from build123d import *

# Parameters (mm, degrees)
SKETCH1_W                  = 70
SKETCH1_H                  = 35
BOSS_EXTRUDE1_DEPTH        = 2
SKETCH2_R                  = 3.75
BOSS_EXTRUDE2_DEPTH        = 8
SKETCH6_W                  = 70
SKETCH6_H                  = 2
BOSS_EXTRUDE3_DEPTH        = 2
F_4_3_4_3_DIAMETER_HOLE1_D = 4.3
CHAMFER1_SIZE              = 0.75
SKETCH5_W                  = 23
SKETCH5_H                  = 14
CUT_EXTRUDE1_DEPTH         = 79.89866919
SKETCH7_W                  = 27
SKETCH7_H                  = 2
SKETCH7_W_2                = 20
BOSS_EXTRUDE4_DEPTH        = 3
SKETCH9_W                  = 27
SKETCH9_H                  = 10
SKETCH9_W_2                = 20
BOSS_EXTRUDE5_DEPTH        = 3
BOSS_EXTRUDE6_DEPTH        = 20
BOSS_EXTRUDE7_START        = -43
BOSS_EXTRUDE7_DEPTH        = 27
CHAMFER3_SIZE              = 0.75
SKETCH11_W                 = 6
SKETCH11_H                 = 10
BOSS_EXTRUDE8_DEPTH        = 10
SKETCH12_R                 = 4.15
CUT_EXTRUDE2_DEPTH         = 5.2
CHAMFER4_SIZE              = 0.4


with BuildPart() as part:
    # Sketch1 → Boss-Extrude1 (new body)
    with BuildSketch(Plane(origin=(0, 0, 0), x_dir=(1, 0, 0), z_dir=(0, 1, 0))):
        with Locations((35, 17.5)):
            Rectangle(SKETCH1_W, SKETCH1_H)
    extrude(amount=BOSS_EXTRUDE1_DEPTH)

    # Sketch2 → Boss-Extrude2 (add)
    with BuildSketch(Plane(origin=(0, 2, 0), x_dir=(1, 0, 0), z_dir=(0, 1, 0))):
        with Locations(Location((66, 31, 0), (0, 0, 90))):
            Circle(SKETCH2_R)
        with Locations(Location((15, 31, 0), (0, 0, 90))):
            Circle(SKETCH2_R)
        with Locations(Location((15, 4, 0), (0, 0, 90))):
            Circle(SKETCH2_R)
        with Locations(Location((66, 4, 0), (0, 0, 90))):
            Circle(SKETCH2_R)
    extrude(amount=BOSS_EXTRUDE2_DEPTH)

    # Sketch6 → Boss-Extrude3 (add)
    with BuildSketch(Plane.XY):
        with Locations((35, 1)):
            Rectangle(SKETCH6_W, SKETCH6_H)
    extrude(amount=BOSS_EXTRUDE3_DEPTH)

    # Ø4.3 (4.3) Diameter Hole1 (through all)
    with Locations(Plane(origin=(0, 10, 0), x_dir=(1, 0, 0), z_dir=(0, 1, 0))):
        with Locations((66, 31), (15, 31), (15, 4), (66, 4)):
            Hole(F_4_3_4_3_DIAMETER_HOLE1_D / 2)

    # Chamfer1
    chamfer1_edges = [part.edges().sort_by_distance(p)[0] for p in [
        (66, 10, -27.25),
        (15, 10, -27.25),
        (15, 10, -0.25),
        (66, 10, -0.25),
    ]]
    chamfer(chamfer1_edges, length=CHAMFER1_SIZE)

    # Sketch5 → Cut-Extrude1 (cut, through all)
    with BuildSketch(Plane.XZ):
        with Locations((38.5, -5)):
            Rectangle(SKETCH5_W, SKETCH5_H)
    extrude(amount=-CUT_EXTRUDE1_DEPTH, mode=Mode.SUBTRACT)

    # Sketch7 → Boss-Extrude4 (add)
    with BuildSketch(Plane.XY.offset(2)):
        with Locations((13.5, 1)):
            Rectangle(SKETCH7_W, SKETCH7_H)
        with Locations((60, 1)):
            Rectangle(SKETCH7_W_2, SKETCH7_H)
    extrude(amount=BOSS_EXTRUDE4_DEPTH)

    # Sketch9 → Boss-Extrude5 (add)
    with BuildSketch(Plane.XY.offset(5)):
        with Locations((13.5, 5)):
            Rectangle(SKETCH9_W, SKETCH9_H)
        with Locations((60, 5)):
            Rectangle(SKETCH9_W_2, SKETCH9_H)
    extrude(amount=BOSS_EXTRUDE5_DEPTH)

    # Sketch10 → Boss-Extrude6 (add)
    with BuildSketch(Plane(origin=(70, 0, 0), x_dir=(0, 0, -1), z_dir=(1, 0, 0))):
        Polygon((-8, 7), (-11, 10), (-11, 0), (-8, 3), align=None)
    extrude(amount=-BOSS_EXTRUDE6_DEPTH)

    # Sketch10<2> → Boss-Extrude7 (add)
    with BuildSketch(Plane(origin=(70, 0, 0), x_dir=(0, 0, -1), z_dir=(1, 0, 0)).offset(BOSS_EXTRUDE7_START)):
        Polygon((-8, 7), (-11, 10), (-11, 0), (-8, 3), align=None)
    extrude(amount=-BOSS_EXTRUDE7_DEPTH)

    # Chamfer3
    chamfer3_edges = [part.edges().sort_by_distance(p)[0] for p in [
        (70, 8.5, 9.5),
        (70, 5, 11),
        (70, 1.5, 9.5),
        (27, 8.5, 9.5),
        (27, 5, 11),
        (27, 1.5, 9.5),
    ]]
    chamfer(chamfer3_edges, length=CHAMFER3_SIZE)

    # Sketch11 → Boss-Extrude8 (add)
    with BuildSketch(Plane.ZY):
        with Locations((8, 5)):
            Rectangle(SKETCH11_W, SKETCH11_H)
    extrude(amount=BOSS_EXTRUDE8_DEPTH)

    # Sketch12 → Cut-Extrude2 (cut)
    with BuildSketch(Plane.XY.offset(11)):
        with Locations((-5, 5)):
            Circle(SKETCH12_R)
    extrude(amount=-CUT_EXTRUDE2_DEPTH, mode=Mode.SUBTRACT)

    # Chamfer4
    chamfer4_edges = [part.edges().sort_by_distance(p)[0] for p in [
        (-9.15, 5, 11),
    ]]
    chamfer(chamfer4_edges, length=CHAMFER4_SIZE)


solid = part.part
Verification items for the finished model (mm, model axes). A direction names the side the tool comes from. Coordinates: 2 decimals unless noted, no trailing zeros. Write each loop counter-clockwise with the first axis right and the second up, starting at its lowest first coordinate (ties: lowest second). Pieces come first, ordered by that corner, then holes. Notation, with made-up numbers: M -18.5,-38.5 L 25.5,-38.5 A23 cw 25.5,-2.5 Z; hole C 46,-6 d10. An arc over 180 degrees is marked long. Use a Markdown table: item, result.
Q1. Sectioned sample at B-B, the plane z = -31. Record the boundary of the cut face in (x, y), plus the area to 3 significant figures.
Reply:
| item | result |
|---|---|
| outline | M 0,0 L 12.85,0 L 12.85,10 L 12,10 L 11.25,9.25 L 11.25,2 L 0,2 Z; M 17.15,0 L 63.85,0 L 63.85,10 L 63,10 L 62.25,9.25 L 62.25,2 L 18.75,2 L 18.75,9.25 L 18,10 L 17.15,10 Z; M 68.15,0 L 70,0 L 70,2 L 69.75,2 L 69.75,9.25 L 69,10 L 68.15,10 Z |
| area | 173 mm² |
Q2. Go/stop test with flat-tipped pins: P1, Ø1.5, axis at y = 2, z = 9.5, coming from the +X side; P2, Ø0.6, axis at x = 44, y = 1, coming from the +Z side; P3, Ø2.5, axis at x = -6, y = 5.5, coming from the +Z side; P4, Ø0.9, axis at y = 8.5, z = 9.5, coming from the +X side. Record where each tip stops, or that it passes through.
Reply:
| item | result |
|---|---|
| P1 | stops at x = 70 |
| P2 | stops at z = -12 |
| P3 | stops at z = 5.8 |
| P4 | stops at x = 69.7 |
Q3. Draft check along Z on faces 1 (the face through (17.282, 5.574, -28.024)), 2 (the face through (70, 1, -7)), 3 (the face through (60, 5, 11)). Enter one of: +Z half, -Z half, draft (parallel to the pull), parting line (faces both ways), or undercut.
Reply:
| item | result |
|---|---|
| face 1 | undercut |
| face 2 | draft |
| face 3 | +Z half |
Q4. Set-up check for faces 4 (the face through (27, 1.6, 3.2)), 5 (the face through (17, 10, -5.3)), 6 (the face through (0, 1, 9)), 7 (the face through (62.282, 5.574, -3.512)): record each of +Z, -Z, +X, -X, +Y, -Y from which the full face is reachable in a straight line by a thin tool's end or side.
Reply:
| item | result |
|---|---|
| face 4 | +Z, +Y, -Y |
| face 5 | +Z, -Z, +X, -X, +Y |
| face 6 | +X, -Y |
| face 7 | +Y |
Q5. Sectioned sample at D-D, the plane z = -10.5. Record the boundary of the cut face in (x, y).
Reply:
| item | result |
|---|---|
| outline | M 0,0 L 27,0 L 27,2 L 0,2 Z; M 50,0 L 70,0 L 70,2 L 50,2 Z |
Q6. Thickness scan on line 1 (Z direction, x = 15, y = 6); line 2 (X direction, y = 3, z = -31); line 3 (X direction, y = 3, z = 7.5). Record the ranges inside material, lowest first.
Reply:
| item | result |
|---|---|
| line 1 | z = -34.75 to -33.15, -28.85 to -27.25, -7.75 to -6.15, -1.85 to -0.25, 5 to 11 |
| line 2 | x = 11.25 to 12.85, 17.15 to 18.75, 62.25 to 63.85, 68.15 to 69.75 |
| line 3 | x = -10 to -8.64, -1.36 to 27, 50 to 70 |
Q7. Sectioned sample at A-A, the plane y = 5. Count the separate pieces of the cut face and the enclosed holes in it, plus the area to 3 significant figures.
Reply:
| item | result |
|---|---|
| separate pieces | 6 |
| enclosed holes | 4 |
| area | 417 mm² |
